```python
from build123d import *

# Parameters (mm, degrees)
SKETCH_1_W          = 105
SKETCH_1_H          = 90
EXTRUDE_1_DEPTH     = 10
SKETCH_3_W          = 5
SKETCH_3_H          = 5
CUT_EXTRUDE_1_DEPTH = 5
SKETCH_4_R          = 1.1
CUT_EXTRUDE_2_DEPTH = 33.2


with BuildPart() as part:
    # 草圖1 → 填料-伸長1 (new body)
    with BuildSketch(Plane.XY):
        with Locations((-6.538461538, -15.192307692)):
            Rectangle(SKETCH_1_W, SKETCH_1_H)
    extrude(amount=EXTRUDE_1_DEPTH)

    # 草圖3 → 除料-伸長1 (cut)
    with BuildSketch(Plane.XY):
        with Locations((43.461538462, -57.692307692)):
            Rectangle(SKETCH_3_W, SKETCH_3_H)
        with Locations((-56.538461538, -57.692307692)):
            Rectangle(SKETCH_3_W, SKETCH_3_H)
        with Locations((43.461538462, 27.307692308)):
            Rectangle(SKETCH_3_W, SKETCH_3_H)
        with Locations((-56.538461538, 27.307692308)):
            Rectangle(SKETCH_3_W, SKETCH_3_H)
    extrude(amount=CUT_EXTRUDE_1_DEPTH, mode=Mode.SUBTRACT)

    # 草圖4 → 除料-伸長2 (cut)
    with BuildSketch(Plane.XY):
        with Locations((-56.538461538, -57.692307692)):
            Circle(SKETCH_4_R)
        with Locations((43.461538462, -57.692307692)):
            Circle(SKETCH_4_R)
        with Locations((43.461538462, 27.307692308)):
            Circle(SKETCH_4_R)
        with Locations((-56.538461538, 27.307692308)):
            Circle(SKETCH_4_R)
    extrude(amount=CUT_EXTRUDE_2_DEPTH, mode=Mode.SUBTRACT)


solid = part.part
```
Model file for the job. Use its own axes, mm. A direction names the side the tool comes from. Give positions to 0.01 mm unless a question says otherwise; leave off trailing zeros.
1) Mould opens along X. For faces 4 (the cylindrical face through (44.51, 27.64, 7.46)), 5 (the flat face through (40.962, 27, 2)), 6 (the flat face through (43, -55.192, 2)) say: +X half, -X half, draft (parallel to the pull), parting line (faces both ways), or undercut.
2) 3-axis set-ups, long thin cutter, end or side, ignore diameter. For faces 1 (the flat face through (42, 27, 5)), 2 (the flat face through (-58, -58, 5)), 3 (the flat face through (-57, 24.808, 2)): which of +Z, -Z, +X, -X, +Y, -Y reach the whole face in a straight line?
3) Pin check, flat tips, straight feed: pin 1 (2.5 mm diameter, centred on y = -56.5, z = 3, fed in from +X); pin 2 (1.5 mm diameter, centred on x = 44.5, y = 26.5, fed in from -Z); pin 3 (1.8 mm diameter, centred on x = 43.46, y = 27.31, fed in from -Z); pin 4 (1.5 mm diameter, centred on x = -57, z = 3, fed in from -Y). Stop position of each tip, or through.
Computed:
1. face 4: undercut
1. face 5: +X half
1. face 6: draft
2. face 1: -Z, +X, +Y
2. face 2: -Z, -X, -Y
2. face 3: -Z, -X, +Y
3. pin 1: stops at x = 40.96
3. pin 2: stops at z = 5
3. pin 3: passes through
3. pin 4: stops at y = -55.19
